Build history of the part. All positions in model axes, mm. A direction names the side the tool comes from. Give positions to 0.01 mm unless a question says otherwise; leave off trailing zeros. Write each loop counter-clockwise with the first axis right and the second up, starting at its lowest first coordinate (ties: lowest second). Pieces come first, ordered by that corner, then holes. Notation, with made-up numbers: (7.25, -38.75) -> (15.25, -38.75) arc R13 ccw to (15.25, -17.75) -> close; hole circle Ø2 at (42.5, 86.5). An arc over 180 degrees is marked (long way). Write item = value, one per line. Start each with the question number.
Q1. Tool access for faces 5 (the face through (-2.8, 1.5, -0.1)), 6 (the face through (0.654, 2.21, -1.112)), 7 (the face through (1.2, 0, 1.2)): list every direction of +Z, -Z, +X, -X, +Y, -Y with a clear straight run to the whole face (end or side of a thin tool).
Q2. Wall check: line 1 (Y direction, x = -1.2, z = -1); line 2 (Z direction, x = 0, y = -10); line 3 (Y direction, x = -0.8, z = -0.4). Give the ranges that are in metal, low to high.
Q3. Saw through at B-B, the plane y = -15. List the corners of the cut face in (x, z).
Q4. Saw through at A-A, the plane z = 0. List the corners of the cut face in (x, y), then the cut area to 3 significant figures.
Q5. Drop flat-ended pins along their axis: P1, Ø3, axis at y = -14, z = -1, coming from the +X side; P2, Ø3, axis at x = -2, z = 1.5, coming from the -Y side; P3, Ø1, axis at y = -12.5, z = 1, coming from the -X side. Give the stop position or say it passes through.
Q6. Mould opens along Z. For faces 1 (the face through (0, -30, 0)), 2 (the face through (0, 1.5, 0)), 3 (the face through (-1.4, -14.74, 0.06)), 4 (the face through (-1.29, 2, 0)) say: pulls with the +Z half, pulls with the -Z half, needs draft (parallel to the pull), parting line crosses it, or undercut.
Q7. Saw through at C-C, the plane z = -1.9. List the corners of the cut face in (x, y), then the cut area to 3 significant figures.
Q8. Saw through at D-D, the plane z = 1.95. List the corners of the cut face in (x, y).
from build123d import *

# Parameters (mm, degrees)
SKETCH_1_R          = 2.8
EXTRUDE_1_DEPTH     = 3
CUT_EXTRUDE_1_DEPTH = 1.5
SKETCH_3_R          = 1.4
EXTRUDE_2_DEPTH     = 30
CHAMFER_1_SIZE      = 0.1


with BuildPart() as part:
    # 草图1 → 凸台-拉伸1 (new body)
    with BuildSketch(Plane(origin=(0, 0, 0), x_dir=(1, 0, 0), z_dir=(0, 1, 0))):
        Circle(SKETCH_1_R)
    extrude(amount=EXTRUDE_1_DEPTH)

    # 草图2 → 切除-拉伸1 (cut)
    with BuildSketch(Plane(origin=(0, 3, 0), x_dir=(1, 0, 0), z_dir=(0, 1, 0))):
        Polygon((0, -1.489563695), (1.29, -0.744781847), (1.29, 0.744781847), (0, 1.489563695), (-1.29, 0.744781847), (-1.29, -0.744781847), align=None)
    extrude(amount=-CUT_EXTRUDE_1_DEPTH, mode=Mode.SUBTRACT)

    # 草图3 → 凸台-拉伸2 (add)
    with BuildSketch(Plane.XZ):
        Circle(SKETCH_3_R)
    extrude(amount=EXTRUDE_2_DEPTH)

    # 倒角1
    chamfer_1_edges = [part.edges().sort_by_distance(p)[0] for p in [
        (-0.645, 3, 1.117172771),
        (0.645, 3, 1.117172771),
        (1.29, 3, 0),
        (0.645, 3, -1.117172771),
        (-0.645, 3, -1.117172771),
        (-1.29, 3, 0),
        (-1.4, -30, 0),
    ]]
    chamfer(chamfer_1_edges, length=CHAMFER_1_SIZE)


solid = part.part
Report:
q1.face_5 = +Y, -Y
q1.face_6 = +Y
q1.face_7 = -Y
q2.line_1 = 0 to 3
q2.line_2 = -1.4 to 1.4
q2.line_3 = -30 to 1.5
q3.outline = circle Ø2.8 at (0, 0)
q4.outline = (-2.8, 0) -> (-1.4, 0) -> (-1.4, -29.9) -> (-1.3, -30) -> (1.3, -30) -> (1.4, -29.9) -> (1.4, 0) -> (2.8, 0) -> (2.8, 3) -> (1.39, 3) -> (1.29, 2.9) -> (1.29, 1.5) -> (-1.29, 1.5) -> (-1.29, 2.9) -> (-1.39, 3) -> (-2.8, 3) -> close
q4.area = 96.9 mm2
q5.P1 = 1.4
q5.P2 = -30
q5.P3 = -1.31
q6.face_1 = needs draft
q6.face_2 = undercut
q6.face_3 = parting line crosses it
q6.face_4 = undercut
q7.outline = (-2.06, 0) -> (2.06, 0) -> (2.06, 3) -> (-2.06, 3) -> close
q7.area = 12.3 mm2
q8.outline = (-2.01, 0) -> (2.01, 0) -> (2.01, 3) -> (-2.01, 3) -> close
